Autodesk Inventor part; units mm, degrees
ref_plane "YZ Plane" through (0, 0, 0) normal (1, 0, 0) x (0, 1, 0)
ref_plane "XZ Plane" through (0, 0, 0) normal (0, 1, 0) x (-1, 0, 0)
ref_plane "XY Plane" through (0, 0, 0) normal (0, 0, 1) x (1, 0, 0)
sketch "スケッチ1" plane through (0, 0, 0) normal (0, 0, 1) x (1, 0, 0)
  circle A0 centre (0, 0) radius 3.6
  dimension "d0" = 7.2
extrude "押し出し1" add sketch "スケッチ1" along normal blind 4
sketch "スケッチ2" plane through (0, 0, 4) normal (0, 0, 1) x (1, 0, 0)
  circle A0 centre (0, 0) radius 2
  dimension "d3" = 4
extrude "押し出し2" add sketch "スケッチ2" along normal blind 15
thread "ねじ1"
sketch "スケッチ3" plane through (0, 0, 0) normal (0, 0, -1) x (-1, 0, 0)
  line L0 (0, -2.0207) -> (-1.75, -1.0104)
  line L1 (-1.75, -1.0104) -> (-1.75, 1.0104)
  line L2 (-1.75, 1.0104) -> (0, 2.0207)
  line L3 (0, 2.0207) -> (1.75, 1.0104)
  line L4 (1.75, 1.0104) -> (1.75, -1.0104)
  line L5 (1.75, -1.0104) -> (0, -2.0207)
  point P0 (0, 0)
  point P1 (0, 0)
  dimension "d8" = 3.5
extrude "押し出し3" cut sketch "スケッチ3" against normal blind 2
properties part number "Bolt_M3_15_for_SetCollar_d6" material "ステンレス鋼"
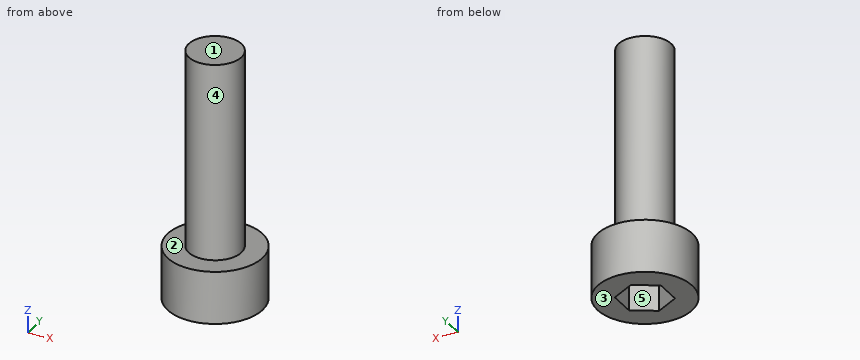
The listing builds one solid part. Answer for the finished solid, in the listing's coordinates (mm). Face numbers are marked on the shaded views. A direction names the side the tool comes from. Give positions to 0.01 mm unless a question says otherwise; leave off trailing zeros. Order: outer loops, then holes, each group sorted by start corner. A loop starts at its lowest first (then second) coordinate and runs counter-clockwise, first axis right, second up. Notation, with made-up numbers: (77.5, 70.25) -> (119.5, 70.25) arc R14 ccw to (119.5, 96.25) -> close; hole circle Ø8 at (58.5, -39). An arc over 180 degrees is marked (long way). Write each question's results on one line, items separated by ' | '.
Q1. The part is cut by section A-A, the plane y = 0. Give the vertices of the cut face in (x, z).
Checked values:
outline: (-3.6, 0) -> (-1.75, 0) -> (-1.75, 2) -> (1.75, 2) -> (1.75, 0) -> (3.6, 0) -> (3.6, 4) -> (2, 4) -> (2, 19) -> (-2, 19) -> (-2, 4) -> (-3.6, 4) -> close
Q2. The part is cut by section D-D, the plane z = 11. Give the vertices of the cut face in (x, y).
Checked values:
outline: circle Ø4 at (0, 0)
Q3. The part is cut by section B-B, the plane x = 1.5. Give the vertices of the cut face in (y, z).
Checked values:
outline: (-3.27, 0) -> (-1.15, 0) -> (-1.15, 2) -> (1.15, 2) -> (1.15, 0) -> (3.27, 0) -> (3.27, 4) -> (1.32, 4) -> (1.32, 19) -> (-1.32, 19) -> (-1.32, 4) -> (-3.27, 4) -> close
Q4. Straight lines are drawn through the part: probe 1 along Z at (x, y) = (0.5, -2.75); probe 2 along Z at (x, y) = (-0.75, 1.5); probe 3 along Y at (x, z) = (0.5, 1.25). For each, find the intervals that lie inside material, in ascending order. Write a range as from..to.
Checked values:
probe 1: z = 0..4 | probe 2: z = 2..19 | probe 3: y = -3.57..-1.73, 1.73..3.57
Q5. The part is cut by section C-C, the plane z = 3. Give the vertices of the cut face in (x, y), and give its area (3 significant figures).
Checked values:
outline: circle Ø7.2 at (0, 0) | area: 40.7 mm^2
Q6. Each of these flat-tipped pins is pushed along its axis until it touches: P1, Ø2, axis at x = -2.5, z = 6, coming from the +Y side; P2, Ø1.5, axis at x = 2.5, z = 7.5, coming from the -Y side; P3, Ø4, axis at x = -1.5, z = 17, coming from the +Y side. Where does it stop, or does it pass through?
Checked values:
P1: stops at y = 1.32 | P2: stops at y = -0.97 | P3: stops at y = 2
Q7. Determine the mould class of the marked faces 3, 4 and 5 for opening direction X: pulls with the +X half, pulls with the -X half, needs draft (parallel to the pull), parting line crosses it, or undercut.
Checked values:
face 3: needs draft | face 4: parting line crosses it | face 5: undercut
Q8. Which of the six approach directions +Z, -Z, +X, -X, +Y, -Y give full straight-line access (tool end or side, diameter ignored) to the marked faces 1 and 2?
Checked values:
face 1: +Z, +X, -X, +Y, -Y | face 2: +Z
